```python
from build123d import *

# Parameters (mm, degrees)
F2_T = -3
F3_R = 1


with BuildPart() as f1:
    # F0 (on Front) → F1 (revolve)
    with BuildSketch(Plane.XZ):
        Polygon((-12.8197669983, 0), (0, 0), (0, 65.9302324057), (-23.5926825553, 65.9302324057), align=None)
    revolve(axis=Axis((0, 0, 32.9651162028), (0, 0, 1)))

    # F2
    f2_openings = [f1.faces().sort_by_distance(p)[0] for p in [
        (0, 0, 65.930232),
    ]]
    offset(amount=F2_T, openings=f2_openings)

    # F3
    f3_edges = [f1.edges().sort_by_distance(p)[0] for p in [
        (23.592683, 0, 65.930232),
        (20.552898, 0, 65.930232),
        (12.819767, 0, 0),
    ]]
    fillet(f3_edges, radius=F3_R)


solid = f1.part
```
Work out the finished part from the listing and answer in its coordinate system (mm). A direction names the side the tool comes from. Give positions to 0.01 mm unless a question says otherwise; leave off trailing zeros. Write each loop counter-clockwise with the first axis right and the second up, starting at its lowest first coordinate (ties: lowest second). Pieces come first, ordered by that corner, then holes. Notation, with made-up numbers: (43.5, 21) -> (57.5, 21) arc R32 ccw to (57.5, 53) -> close; hole circle Ø11 at (-23, 48). An arc over 180 degrees is marked (long way). Write item = value, one per line.
Q1. A tool of negligible diameter and unlimited length cuts with its end or side. For faces 4 (the flat face through (0, 0, 3)), 5 (the flat face through (0, 0, 0)), from which of +Z, -Z, +X, -X, +Y, -Y can it reach the whole face along a straight path? Write none if from no direction.
Computed values:
face_4 = +Z
face_5 = -Z, +X, -X, +Y, -Y
Q2. For a pull along X with two mould halves and no side action, classify faces 1 (the conical face through (12.12, 9.29, 33.61)), 2 (the conical face through (3.925, 17.676, 32.356)), 3 (the flat face through (12, 18, 65.93)) as pulls with the +X half, pulls with the -X half, needs draft (parallel to the pull), parting line crosses it, or undercut.
Computed values:
face_1 = undercut
face_2 = parting line crosses it
face_3 = needs draft
Q3. Flat-ended cylindrical pins translate along their axes: pin 1 Ø5 at (y, z) = (-3, 35.5) entering from -X; pin 2 Ø6 at (x, z) = (-6, 8) entering from -Y; pin 3 Ø10.5 at (x, y) = (1.5, 4) entering from +Z. Find the tip coordinate at first contact, or state that the pin passes through.
Computed values:
pin_1 = -18.89
pin_2 = -13.97
pin_3 = 3
Q4. Section C-C on z = 43 is taken. Determine the outline of the cut face in (x, y), and give its area (3 significant figures).
Computed values:
outline = circle Ø39.69 at (0, 0); hole circle Ø33.61 at (0, 0)
area = 350 mm^2
Q5. Consider line 1 along Z through (x, y) = (2, -10); line 2 along Y through (x, z) = (-5.5, 23.5); line 3 along Y through (x, z) = (16, 56). Determine where each line is inside the solid, lowest interval first.
Computed values:
line_1 = 0 to 3
line_2 = -15.73 to -12.46, 12.46 to 15.73
line_3 = -15.06 to -10.12, 10.12 to 15.06
Q6. Section A-A on y = 0 is taken. Determine the outline of the cut face in (x, z).
Computed values:
outline = (-23.4, 64.77) -> (-12.96, 0.84) arc R1 ccw to (-11.97, 0) -> (11.97, 0) arc R1 ccw to (12.96, 0.84) -> (23.4, 64.77) arc R1 ccw to (22.42, 65.93) -> (21.4, 65.93) arc R1 ccw to (20.42, 65.09) -> (10.27, 3) -> (-10.27, 3) -> (-20.42, 65.09) arc R1 ccw to (-21.4, 65.93) -> (-22.42, 65.93) arc R1 ccw to start
Q7. Section D-D on z = 18 is taken. Determine the outline of the cut face in (x, y), and give its area (3 significant figures).
Computed values:
outline = circle Ø31.52 at (0, 0); hole circle Ø25.44 at (0, 0)
area = 272 mm^2
